Input: part model. Units: mm. Frame: model coordinates. Face numbers are marked on the shaded views. A direction names the side the tool comes from. Give positions to 0.01 mm unless a question says otherwise; leave off trailing zeros. Loops run counter-clockwise (first coordinate to the right, second up) from the corner with the lowest first, then second, coordinate; pieces in that order, holes last. Notation, with made-up numbers: (16, -0.75) -> (53, -0.75) arc R31 cw to (53, 23.25) -> close; hole circle Ø7 at (-25, -1.5). An arc over 180 degrees is marked (long way). One line per question, with ' | ' between items.
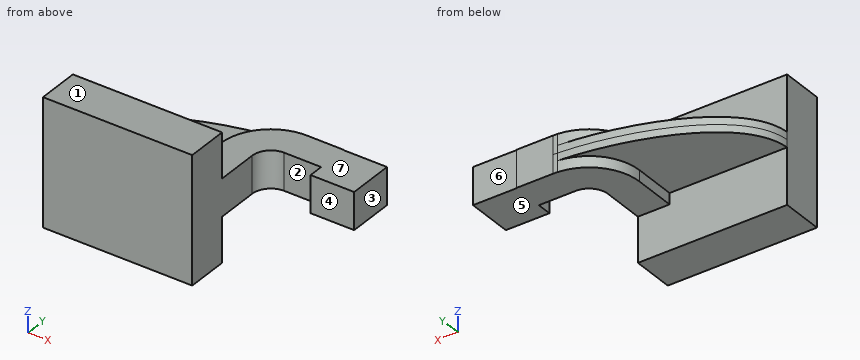
from build123d import *

# Parameters (mm, degrees)
F1_DEPTH = 42.4
F0_W     = 29.2045593262
F0_H     = 20.9105454808
F0_H_2   = 9.8793879763
F2_DEPTH = 12.4
F3_DEPTH = 5


with BuildPart() as f1:
    # F0 (on Top) → F1 (new body, symmetric)
    with BuildSketch(Plane.XY):
        Polygon((-50, -14), (50, -14), (50, 14), (28.8000002503, 14), (-50, 14), align=None)
    extrude(amount=F1_DEPTH, both=True)

    # F0 (on Top) → F2 (join, symmetric)
    with BuildSketch(Plane.XY):
        with BuildLine():
            Line((28.8000002503, 14), (50, 14))
            Line((50, 14), (50, 42.2444418685))
            ThreePointArc((50, 42.2444418685), (53.6694869302, 51.1033669823), (62.528412044, 54.7728539125))
            Line((62.528412044, 54.7728539125), (87.2514024377, 54.7728539125))
            Line((87.2514024377, 54.7728539125), (87.2514024377, 75.6833993933))
            Line((87.2514024377, 75.6833993933), (87.2514024377, 75.9728536622))
            Line((87.2514024377, 75.9728536622), (62.528412044, 75.9728536622))
            add(Edge.make_bspline(
                [(59.6423828035, 75.8491528083), (60.623221152, 75.9014989859), (61.5857310507, 75.9427206922), (62.528412044, 75.9728536622)],
                knots=[125.3288073091, 125.3288073091, 125.3288073091, 125.3288073091, 128.4650851718, 128.4650851718, 128.4650851718, 128.4650851718], degree=3))
            ThreePointArc((59.6423828035, 75.8491528083), (37.6793985345, 65.0508508301), (28.8000002503, 42.2444418685))
            Line((28.8000002503, 42.2444418685), (28.8000002503, 14))
        make_face()
        with Locations((101.8536821008, 65.2281266529)):
            Rectangle(F0_W, F0_H)
        with Locations((101.8536821008, 49.8331599243)):
            Rectangle(F0_W, F0_H_2)
    extrude(amount=F2_DEPTH, both=True)

    # F0 (on Top) → F3 (join, symmetric)
    with BuildSketch(Plane.XY):
        with BuildLine():
            add(Edge.make_bspline(
                [(-50, 14), (-48.0165507364, 53.9010766579), (20.4470991711, 73.7573470777), (59.6423828035, 75.8491528083)],
                knots=[0, 0, 0, 0, 125.3288073091, 125.3288073091, 125.3288073091, 125.3288073091], degree=3))
            Line((-50, 14), (28.8000002503, 14))
            Line((28.8000002503, 14), (28.8000002503, 42.2444418685))
            ThreePointArc((28.8000002503, 42.2444418685), (37.6793985345, 65.0508508301), (59.6423828035, 75.8491528083))
        make_face()
    extrude(amount=F3_DEPTH, both=True)


solid = f1.part
1. Section query B-B (x = 93). Output: boundary loops of the cut face in (y, z).
Determined:
outline: (44.89, -12.4) -> (75.68, -12.4) -> (75.68, 12.4) -> (44.89, 12.4) -> close
2. Pull-direction query (X, two-part tool) for the marked faces 1, 2 and 3; classes: pulls with the +X half, pulls with the -X half, needs draft (parallel to the pull), parting line crosses it, or undercut.
Determined:
face 1: needs draft | face 2: undercut | face 3: pulls with the +X half
3. Ray query, line 1 along X through (y, z) = (27, 5.5); line 2 along Z through (x, y) = (20.5, 68); line 3 along X through (y, z) = (-3, 33). Return the intervals inside material, ascending. Write a range as from..to.
Determined:
line 1: x = 28.8..50 | line 2: z = -5..5 | line 3: x = -50..50
4. Pin query (flat end, axial travel): P1, Ø1, axis at x = 44.5, z = 32.5, coming from the +Y side; P2, Ø5, axis at x = 55, y = 47, coming from the -Z side; P3, Ø1.5, axis at x = -14.5, y = 32.5, coming from the -Z side; P4, Ø11, axis at y = 49, z = -2, coming from the -X side. Return the tip coordinate at first contact, or that it passes through.
Determined:
P1: stops at y = 14 | P2: passes through | P3: stops at z = -5 | P4: stops at x = -34.08
5. Section query A-A (z = 26.5). Output: boundary loops of the cut face in (x, y).
Determined:
outline: (-50, -14) -> (50, -14) -> (50, 14) -> (-50, 14) -> close
6. Reachability of the marked faces 4, 5, 6 and 7 from +Z, -Z, +X, -X, +Y, -Y: full face, straight path, thin tool, end or side. Return the list, or none.
Determined:
face 4: +Z, -Z, +X, -Y | face 5: -Z, +X, -X, +Y | face 6: +Z, -Z, +X, +Y | face 7: +Z, +X, -X, +Y
